For this review, take the finished solid that the model builds, in its own axes (mm). A direction names the side the tool comes from. Coordinates: 2 decimals unless noted, no trailing zeros. Answer as a JSON object with one key per item and string values. Group by question number.
Item 1: Mouldability with a two-part tool opening along X and no side actions: class faces 1 (the face through (-1, -15, -33)), 2 (the face through (-0.04, 7.81, -1.73)), 3 (the face through (-3, 8.3, 0.6)) as +X half, -X half, draft (parallel to the pull), parting line (faces both ways), or undercut.
Item 2: Wall thickness on L1, parallel to Y at x = 0.85, z = 0; L2, parallel to Y at x = 1.2, z = 5 (3 decimals); L3, parallel to Z at x = 1.1, y = 5 (3 decimals): over which ranges is each line inside the solid? List them lowest first. Write a range as from..to.
Item 3: Insertion check: pin 1 (13 mm diameter, centred on y = 0, z = 0, fed in from +X). The pin has a flat end and moves straight along its axis. Give the tip position at first contact, or say it passes through.
Item 4: Tool access review of faces 4 (the face through (1, -15, 33)), 5 (the face through (3, 8.3, -0.6)): name each direction out of +Z, -Z, +X, -X, +Y, -Y from which nothing blocks a thin tool from reaching the whole face with its end or side.
from build123d import *

# Parameters (mm, degrees)
CONG_1_R = 1


with BuildPart() as part:
    # Esquisse1 → Révolution2 (revolve)
    with BuildSketch(Plane.XY, mode=Mode.PRIVATE) as r_volution2_sk:
        Polygon((-1, 36), (1, 36), (1, 41), (3, 41), (3, 8), (-3, 8), (-3, 41), (-1, 41), align=None)
    revolve(r_volution2_sk.sketch.rotate(Axis((0, 0, 0), (1, 0, 0)), 90), axis=Axis((0, 0, 0), (1, 0, 0)))

    # Congé1
    cong_1_edges = [part.edges().sort_by_distance(p)[0] for p in [
        (-3, 0, -41),
        (-1, 0, -41),
        (1, 0, -41),
        (3, 0, -41),
    ]]
    fillet(cong_1_edges, radius=CONG_1_R - 0.0001)  # a hair under: the kernel refuses the full size


solid = part.part
From the geometry:
{
 "1": {"face 1": "undercut", "face 2": "draft", "face 3": "-X half"},
 "2": {"L1": "y = -36..-8, 8..36", "L2": "y = -40.291..-6.245, 6.245..40.291", "L3": "z = -40.126..-6.245, 6.245..40.126"},
 "3": {"pin 1": "passes through"},
 "4": {"face 4": "none", "face 5": "+Z, -Z, +X, +Y, -Y"}
}
